```python
from build123d import *

# Parameters (mm, degrees)
FASE1_SIZE = 0.2


with BuildPart() as part:
    # Skizze2 → Rotation2 (revolve)
    with BuildSketch(Plane(origin=(0, 0, 0), x_dir=(0, 0, -1), z_dir=(1, 0, 0))):
        Polygon((-12.5, 2), (-12.5, -2), (-11.85, -2), (-11.85, -1.75), (-10.65, -1.75), (-10.65, -2), (-10, -2), (-10, 2), (-10.65, 2), (-10.65, 1.75), (-11.85, 1.75), (-11.85, 2), align=None)
    revolve(axis=Axis((0, -18.122913865, 0), (0, 1, 0)))

    # Fase1
    fase1_edges = [part.edges().sort_by_distance(p)[0] for p in [
        (0, 2, -10),
        (0, -2, -10),
        (0, -2, -12.5),
        (0, 2, -12.5),
    ]]
    chamfer(fase1_edges, length=FASE1_SIZE)


solid = part.part
```
Here's how the part is built. I have some questions about the finished solid (model axes, mm). A direction names the side the tool comes from. Coordinates: 2 decimals unless noted, no trailing zeros. Loops run counter-clockwise (first coordinate to the right, second up) from the corner with the lowest first, then second, coordinate; pieces in that order, holes last. Notation, with made-up numbers: (-11, -28.75) -> (32, -28.75) arc R30 cw to (32, 5.25) -> close; hole circle Ø3 at (66.5, -5.75). An arc over 180 degrees is marked (long way). Return JSON: item names as keys, results as strings.
1) Thinking about a two-plate mould opening in Z: for faces 1 (the face through (3.755, -0.025, 11.923)), 2 (the face through (2, -1.75, -11)), 3 (the face through (11, -2, -5)), which applies, +Z half, -Z half, draft (parallel to the pull), parting line (faces both ways), or undercut?
Results below:
{"face 1": "parting line", "face 2": "undercut", "face 3": "draft"}
2) Will these pins go through, and if not, where does the flat tip stop? pin 1 (1.5 mm diameter, centred on x = -7.5, y = 0, fed in from +Z); pin 2 (6 mm diameter, centred on x = -0.5, z = -7.5, fed in from +Y); pin 3 (1.5 mm diameter, centred on y = 1, z = -4.5, fed in from -X); pin 4 (2 mm diameter, centred on y = 1.5, z = -6, fed in from -X).
Results below:
{"pin 1": "z = 10.52", "pin 2": "y = 2", "pin 3": "x = -11.92", "pin 4": "x = -11.46"}
3) For faces 4 (the face through (-9.76, 0.03, -2.17)), 5 (the face through (2, 1.75, 11)), which set-ups out of +Z, -Z, +X, -X, +Y, -Y let a thin tool reach every point of the face, with its end or its side?
Results below:
{"face 4": "+Y, -Y", "face 5": "+Y"}
4) If we section it at C-C, the plane y = -1.25: Write out the boundary of the cut face in (x, z).
Results below:
{"outline": "circle Ø25 at (0, 0); hole circle Ø20 at (0, 0)"}
5) I need wall thicknesses on line 1 (X direction, y = 0.8, z = 0); line 2 (X direction, y = 1.95, z = 0). Which ranges of each line are inside material? Lowest first, please. Write a range as from..to.
Results below:
{"line 1": "-12.5..-10, 10..12.5", "line 2": "-12.35..-11.85, -10.65..-10.15, 10.15..10.65, 11.85..12.35"}
